Read the model definition and answer for the solid it produces. Units are mm, in the model's axes. A direction names the side the tool comes from. Give positions to 0.01 mm unless a question says otherwise; leave off trailing zeros. Loops run counter-clockwise (first coordinate to the right, second up) from the corner with the lowest first, then second, coordinate; pieces in that order, holes last.
(1) Which of the six approach directions +Z, -Z, +X, -X, +Y, -Y give full straight-line access (tool end or side, diameter ignored) to faces 4 (the face through (7.11, -5.66, 0.76)), 5 (the face through (-4, 5, 0)), 6 (the face through (3.105, 10.782, 0.76))?
(2) Find section B-B, the plane y = 0.5. Write down the section's boundary in (x, z), then the cut area to 3 significant figures.
(3) Find section C-C, the plane y = 9.25. Write down the section's boundary in (x, z).
(4) Find section A-A, the plane x = -6. Write down the section's boundary in (y, z), then the cut area to 3 significant figures.
(5) Find section D-D, the plane x = -11. Write down the section's boundary in (y, z).
(6) Straight lines are drawn through the part: probe 1 along Y at (x, z) = (-1, 0.65); probe 2 along X at (y, z) = (0, 1.4); probe 3 along Y at (x, z) = (7, 0.2). For each, find the intervals that lie inside material, in ascending order.
(7) Determine the mould class of faces 1 (the face through (15.71, -6.75, 0.76)), 2 (the face through (11.213, -5.639, 0.76)), 3 (the face through (16.012, 2, 1)) for opening direction Y: pulls with the +Y half, pulls with the -Y half, needs draft (parallel to the pull), parting line crosses it, or undercut.
```python
from build123d import *

# Parameters (mm, degrees)
SKETCH_1_W          = 40
SKETCH_1_H          = 18.871619184
SKETCH_1_R          = 1.1
EXTRUDE_1_DEPTH     = 1.5
SKETCH_2_W          = 20.265588098
SKETCH_2_H          = 7.002088202
CUT_EXTRUDE_1_DEPTH = 1.5
FILLET_1_R          = 1
FILLET_2_R          = 1
FILLET_3_R          = 2


with BuildPart() as part:
    # 草图1 → 凸台-拉伸1 (new body)
    with BuildSketch(Plane.XY):
        with Locations((-3.988440653, 2.400990099)):
            Rectangle(SKETCH_1_W, SKETCH_1_H)
        with Locations((-21.738440653, 9.900990099)):
            Circle(SKETCH_1_R, mode=Mode.SUBTRACT)
        with Locations((-21.738440653, -5.099009901)):
            Circle(SKETCH_1_R, mode=Mode.SUBTRACT)
        with Locations((13.761559347, -5.099009901)):
            Circle(SKETCH_1_R, mode=Mode.SUBTRACT)
        with Locations((13.761559347, 9.900990099)):
            Circle(SKETCH_1_R, mode=Mode.SUBTRACT)
    extrude(amount=EXTRUDE_1_DEPTH)

    # 草图2 → 切除-拉伸1 (cut)
    with BuildSketch(Plane.XY.offset(1.5)):
        Polygon((-16.728608447, 11.836799691), (-14.639805099, 9.747996342), (2.071462084, 9.747996342), (5.519738876, 13.196273134), (-14.871851344, 13.196273134), align=None)
        with Locations((-0.480960338, 0.9646533)):
            Rectangle(SKETCH_2_W, SKETCH_2_H)
        with BuildLine():
            Line((-16.310435566, -5.15021554), (-13.288801442, -5.15021554))
            ThreePointArc((-13.288801442, -5.15021554), (-12.788801442, -5.65021554), (-13.288801442, -6.15021554))
            Line((-13.288801442, -6.15021554), (-16.310435566, -6.15021554))
            ThreePointArc((-16.310435566, -6.15021554), (-16.810435566, -5.65021554), (-16.310435566, -5.15021554))
        make_face()
        with BuildLine():
            Line((7.610434302, -5.15021554), (10.713575026, -5.15021554))
            ThreePointArc((10.713575026, -5.15021554), (11.213575026, -5.65021554), (10.713575026, -6.15021554))
            Line((10.713575026, -6.15021554), (7.610434302, -6.15021554))
            ThreePointArc((7.610434302, -6.15021554), (7.110434302, -5.65021554), (7.610434302, -5.15021554))
        make_face()
    extrude(amount=-CUT_EXTRUDE_1_DEPTH, mode=Mode.SUBTRACT)

    # 圆角1
    fillet_1_edges = [part.edges().sort_by_distance(p)[0] for p in [
        (4.160265432, 11.836799691, 0.75),
        (-16.728608447, 11.836799691, 0.75),
        (2.071462084, 9.747996342, 0.75),
        (-14.639805099, 9.747996342, 0.75),
    ]]
    fillet(fillet_1_edges, radius=FILLET_1_R)

    # 圆角2
    fillet_2_edges = [part.edges().sort_by_distance(p)[0] for p in [
        (16.011559347, -7.034819493, 0.75),
        (-23.988440653, -7.034819493, 0.75),
        (-23.988440653, 11.836799691, 0.75),
        (16.011559347, 11.836799691, 0.75),
    ]]
    fillet(fillet_2_edges, radius=FILLET_2_R)

    # 圆角3
    fillet_3_edges = [part.edges().sort_by_distance(p)[0] for p in [
        (9.651833711, 4.465697401, 0.75),
        (9.651833711, -2.536390801, 0.75),
        (-10.613754387, -2.536390801, 0.75),
        (-10.613754387, 4.465697401, 0.75),
    ]]
    fillet(fillet_3_edges, radius=FILLET_3_R)


solid = part.part
```
Entries:
1. face 4: +Z, -Z
1. face 5: -Z, +X, -X, +Y, -Y
1. face 6: +Z, -Z, +Y
2. outline: (-23.99, 0) - (-10.61, 0) - (-10.61, 1.5) - (-23.99, 1.5) - close; (9.65, 0) - (16.01, 0) - (16.01, 1.5) - (9.65, 1.5) - close
2. area: 29.6 mm2
3. outline: (-23.99, 0) - (-22.63, 0) - (-22.63, 1.5) - (-23.99, 1.5) - close; (-20.85, 0) - (12.87, 0) - (12.87, 1.5) - (-20.85, 1.5) - close; (14.65, 0) - (16.01, 0) - (16.01, 1.5) - (14.65, 1.5) - close
4. outline: (-7.03, 0) - (-2.54, 0) - (-2.54, 1.5) - (-7.03, 1.5) - close; (4.47, 0) - (9.75, 0) - (9.75, 1.5) - (4.47, 1.5) - close
4. area: 14.7 mm2
5. outline: (-7.03, 0) - (9.75, 0) - (9.75, 1.5) - (-7.03, 1.5) - close
6. probe 1: y = -7.03 to -2.54, 4.47 to 9.75
6. probe 2: x = -23.99 to -10.61, 9.65 to 16.01
6. probe 3: y = -7.03 to -2.54, 4.47 to 11.84
7. face 1: pulls with the -Y half
7. face 2: undercut
7. face 3: needs draft
